Design review of the part built by this model. Coordinates are the model's own, in mm. A direction names the side the tool comes from. Coordinates: 2 decimals unless noted, no trailing zeros. Loops run counter-clockwise (first coordinate to the right, second up) from the corner with the lowest first, then second, coordinate; pieces in that order, holes last. Notation, with made-up numbers: (4.5, 54) - (40.5, 54) arc R31 ccw to (40.5, 93) - close; hole circle Ø7 at (0, 61). An arc over 180 degrees is marked (long way). Use one line per item in the form item = value. Start each with the question number.
(1) Clearance check with flat-ended pins moving along their axes: pin 1 Ø1.4 at (x, y) = (59.5, -1) entering from +Z; pin 2 Ø3 at (y, z) = (9, -5) entering from +X (3 decimals); pin 3 Ø4 at (x, z) = (60.5, -3) entering from -Y. State where each tip first meets the part, or that it passes through.
(2) Add section B-B (z = -4.25). State the section outline as (x, y) points (3 decimals).
(3) For L1, parallel to Z at x = -50, y = -2.5; L2, parallel to Y at x = -48, z = 2.5; L3, parallel to X at y = 6, z = 2 (3 decimals), list the stretches that pass through material, from the lowest coordinate up.
(4) The part is to be moulded in two halves that separate along Y. For faces 4 (the face through (-53, -13.578, 0)), 5 (the face through (62.375, -3, 0)), 6 (the face through (-1, -18.078, 0)), say which applies: pulls with the +Y half, pulls with the -Y half, needs draft (parallel to the pull), parting line crosses it, or undercut.
(5) Add section C-C (y = 8.25). State the section outline as (x, z) points (3 decimals).
(6) Add section A-A (y = -0.75). State the section outline as (x, z) points (3 decimals).
(7) Tool access review of faces 1 (the face through (60, 6.922, 0)), 2 (the face through (-53, 6.922, 0)), 3 (the face through (60, -13.078, 0)): name each direction out of +Z, -Z, +X, -X, +Y, -Y from which nothing blocks a thin tool from reaching the whole face with its end or side.
(8) Add section D-D (z = -12). State the section outline as (x, y) points (3 decimals).
```python
from build123d import *

# Parameters (mm, degrees)
SKETCH1_W           = 115.25
SKETCH1_H           = 30
BOSS_EXTRUDE1_DEPTH = 15
SKETCH2_W           = 20.5
SKETCH2_H           = 20.5
CUT_EXTRUDE2_DEPTH  = 10
SKETCH3_W           = 20
SKETCH3_H           = 20
BOSS_EXTRUDE2_DEPTH = 4.75


with BuildPart() as part:
    # Sketch1 → Boss-Extrude1 (new, symmetric)
    with BuildSketch(Plane.XY):
        with Locations((0, -3.077586207)):
            Rectangle(SKETCH1_W, SKETCH1_H)
    extrude(amount=BOSS_EXTRUDE1_DEPTH, both=True)

    # Sketch2 → Cut-Extrude2 (cut)
    with BuildSketch(Plane.ZY.offset(57.625)):
        with Locations((0, -3.327586207)):
            Rectangle(SKETCH2_W, SKETCH2_H)
    extrude(amount=-CUT_EXTRUDE2_DEPTH, mode=Mode.SUBTRACT)

    # Sketch3 → Boss-Extrude2 (add)
    with BuildSketch(Plane(origin=(57.625, 0, 0), x_dir=(0, 0, -1), z_dir=(1, 0, 0))):
        with Locations((0, -3.077586207)):
            Rectangle(SKETCH3_W, SKETCH3_H)
    extrude(amount=BOSS_EXTRUDE2_DEPTH)


solid = part.part
```
Computed values:
q1.pin_1 = 10
q1.pin_2 = 57.625
q1.pin_3 = -13.08
q2.outline = (-57.625, -18.078) - (57.625, -18.078) - (57.625, -13.078) - (62.375, -13.078) - (62.375, 6.922) - (57.625, 6.922) - (57.625, 11.922) - (-57.625, 11.922) - (-57.625, 6.922) - (-47.625, 6.922) - (-47.625, -13.578) - (-57.625, -13.578) - close
q3.L1 = -15 to -10.25, 10.25 to 15
q3.L2 = -18.08 to -13.58, 6.92 to 11.92
q3.L3 = -47.625 to 62.375
q4.face_4 = undercut
q4.face_5 = needs draft
q4.face_6 = pulls with the -Y half
q5.outline = (-57.625, -15) - (57.625, -15) - (57.625, 15) - (-57.625, 15) - close
q6.outline = (-57.625, -15) - (57.625, -15) - (57.625, -10) - (62.375, -10) - (62.375, 10) - (57.625, 10) - (57.625, 15) - (-57.625, 15) - (-57.625, 10.25) - (-47.625, 10.25) - (-47.625, -10.25) - (-57.625, -10.25) - close
q7.face_1 = +Z, -Z, +X, +Y
q7.face_2 = -X
q7.face_3 = +Z, -Z, +X, -Y
q8.outline = (-57.625, -18.078) - (57.625, -18.078) - (57.625, 11.922) - (-57.625, 11.922) - close
